from build123d import *

# Parameters (mm, degrees)
BOSS_EXTRUDE1_DEPTH = 45
SKETCH2_W           = 15
SKETCH2_H           = 10
BOSS_EXTRUDE2_DEPTH = 15
CUT_EXTRUDE1_START  = -35
SKETCH3_R           = 3.25
CUT_EXTRUDE1_DEPTH  = 35
SKETCH4_W           = 35
SKETCH4_H           = 5
BOSS_EXTRUDE3_DEPTH = 10
FILLET1_R           = 2


with BuildPart() as part:
    # Sketch1 → Boss-Extrude1 (new body)
    with BuildSketch(Plane(origin=(0, 0, 0), x_dir=(1, 0, 0), z_dir=(0, 1, 0))):
        Polygon((-17.5, 7.5), (-7.5, 7.5), (-7.5, -7.5), (7.5, -7.5), (7.5, 7.5), (17.5, 7.5), (17.5, -17.5), (-17.5, -17.5), align=None)
    extrude(amount=BOSS_EXTRUDE1_DEPTH)

    # Sketch2 → Boss-Extrude2 (add)
    with BuildSketch(Plane(origin=(0, 0, 7.5), x_dir=(-1, 0, 0), z_dir=(0, 0, -1))):
        with Locations((0, 40)):
            Rectangle(SKETCH2_W, SKETCH2_H)
        with Locations((0, 15)):
            Rectangle(SKETCH2_W, SKETCH2_H)
    extrude(amount=BOSS_EXTRUDE2_DEPTH)

    # Sketch3 → Cut-Extrude1 (cut)
    with BuildSketch(Plane(origin=(0, 45, 0), x_dir=(1, 0, 0), z_dir=(0, 1, 0)).offset(CUT_EXTRUDE1_START)):
        with Locations(Location((0, 0, 0), (0, 0, 270))):
            Circle(SKETCH3_R)
    extrude(amount=CUT_EXTRUDE1_DEPTH, mode=Mode.SUBTRACT)

    # Sketch4 → Boss-Extrude3 (add)
    with BuildSketch(Plane(origin=(0, 0, -7.5), x_dir=(-1, 0, 0), z_dir=(0, 0, -1))):
        with Locations((0, 42.5)):
            Rectangle(SKETCH4_W, SKETCH4_H)
    extrude(amount=BOSS_EXTRUDE3_DEPTH)

    # Fillet1
    fillet1_edges = [part.edges().sort_by_distance(p)[0] for p in [
        (17.5, 22.5, 17.5),
        (-17.5, 22.5, 17.5),
        (0, 45, 17.5),
    ]]
    fillet(fillet1_edges, radius=FILLET1_R)


solid = part.part
Could you check a few things on this model? Use its own coordinates, in mm. A direction names the side the tool comes from. Give positions to 0.01 mm unless a question says otherwise; leave off trailing zeros. Loops run counter-clockwise (first coordinate to the right, second up) from the corner with the lowest first, then second, coordinate; pieces in that order, holes last. Notation, with made-up numbers: M 82.25,-37.5 L 125.25,-37.5 A33 cw 125.25,-6.5 Z; hole C 76,82.5 d6. An arc over 180 degrees is marked long. Answer as a JSON object with one key per item and string values.
Q1. Suppose I cut it at D-D, the plane z = 6. List the corners of the cut face in (x, y) for me.
Values found:
{"outline": "M -17.5,0 L -7.5,0 L -7.5,10 L 7.5,10 L 7.5,0 L 17.5,0 L 17.5,45 L -17.5,45 Z; hole M -7.5,20 L 7.5,20 L 7.5,35 L -7.5,35 Z"}
Q2. Suppose I cut it at C-C, the plane y = 31. List the corners of the cut face in (x, z) for me, plus the area to 3 significant figures.
Values found:
{"outline": "M -17.5,-7.5 L -7.5,-7.5 L -7.5,7.5 L 7.5,7.5 L 7.5,-7.5 L 17.5,-7.5 L 17.5,15.5 A2 ccw 15.5,17.5 L -15.5,17.5 A2 ccw -17.5,15.5 Z", "area": "648 mm²"}
Q3. If we mould it in two halves opening along Y, with no side actions, what happens to faces 1 (the cylindrical face through (-0.25, 44.4, 16.93)), 2 (the flat face through (0, 21, 17.5)), 3 (the flat face through (0, 27, 7.5))? For each: pulls with the +Y half, pulls with the -Y half, needs draft (parallel to the pull), parting line crosses it, or undercut.
Values found:
{"face 1": "pulls with the +Y half", "face 2": "needs draft", "face 3": "undercut"}
Q4. Suppose I cut it at B-B, the plane z = 0. List the corners of the cut face in (x, y) for me.
Values found:
{"outline": "M -17.5,0 L -7.5,0 L -7.5,10 L -3.25,10 L -3.25,20 L -7.5,20 L -7.5,35 L -3.25,35 L -3.25,45 L -17.5,45 Z; M 3.25,10 L 7.5,10 L 7.5,0 L 17.5,0 L 17.5,45 L 3.25,45 L 3.25,35 L 7.5,35 L 7.5,20 L 3.25,20 Z"}
Q5. Suppose I cut it at A-A, the plane x = 0. List the corners of the cut face in (y, z) for me, plus the area to 3 significant figures.
Values found:
{"outline": "M 0,7.5 L 10,7.5 L 10,3.25 L 20,3.25 L 20,7.5 L 35,7.5 L 35,3.25 L 45,3.25 L 45,15.5 A2 ccw 43,17.5 L 0,17.5 Z; M 10,-7.5 L 20,-7.5 L 20,-3.25 L 10,-3.25 Z; M 35,-7.5 L 40,-7.5 L 40,-17.5 L 45,-17.5 L 45,-3.25 L 35,-3.25 Z", "area": "669 mm²"}
Q6. If I drill on probe 1 along Y at (x, z) = (-1, 6); probe 2 along X at (y, z) = (6, 4); probe 3 along Z at (x, y) = (0, 17.25), over which ranges is the centre line in solid material (lowest first)? Write a range as [from, to].
Values found:
{"probe 1": "y = [10, 20], [35, 45]", "probe 2": "x = [-17.5, -7.5], [7.5, 17.5]", "probe 3": "z = [-7.5, -3.25], [3.25, 17.5]"}
Q7. For P1, Ø16.5, axis at x = -2, y = 27.5, coming from the -Z side; P2, Ø3, axis at x = 1.5, z = -12.5, coming from the -Y side; P3, Ø10, axis at y = 21, z = -13.5, coming from the +X side; P4, Ø16.5, axis at x = 1, z = -1, coming from the -Y side, each with a flat end and sliding along its axis, tell me the tip position at first contact or that it passes through.
Values found:
{"P1": "stops at z = -7.5", "P2": "stops at y = 40", "P3": "passes through", "P4": "stops at y = 0"}
Q8. For faces 4 (the flat face through (17.5, 22, 3)), 5 (the flat face through (0, 40, -12)), 6 (the flat face through (-7.5, 5, 0)), 7 (the flat face through (-7.5, 27, 0)), 8 (the cylindrical face through (-1.978, 39.93, -2.579)), which set-ups out of +Z, -Z, +X, -X, +Y, -Y let a thin tool reach every point of the face, with its end or its side?
Values found:
{"face 4": "+Z, -Z, +X, +Y, -Y", "face 5": "-Z, +X, -X, -Y", "face 6": "-Z, -Y", "face 7": "-Z", "face 8": "+Y, -Y"}
